Job drawing, mm, ordinate dimensions from the low corner. One solid piece. A direction names the side the tool comes from. Give positions to 0.01 mm unless a question says otherwise; leave off trailing zeros. Order: outer loops, then holes, each group sorted by start corner. A loop starts at its lowest first (then second) coordinate and runs counter-clockwise, first axis right, second up. Notation, with made-up numbers: (80, 40.25) - (101, 40.25) arc R26 ccw to (101, 67.25) - close; hole circle Ø7 at (48.5, 19). An arc over 180 degrees is marked (long way). One line per item, written item: value.
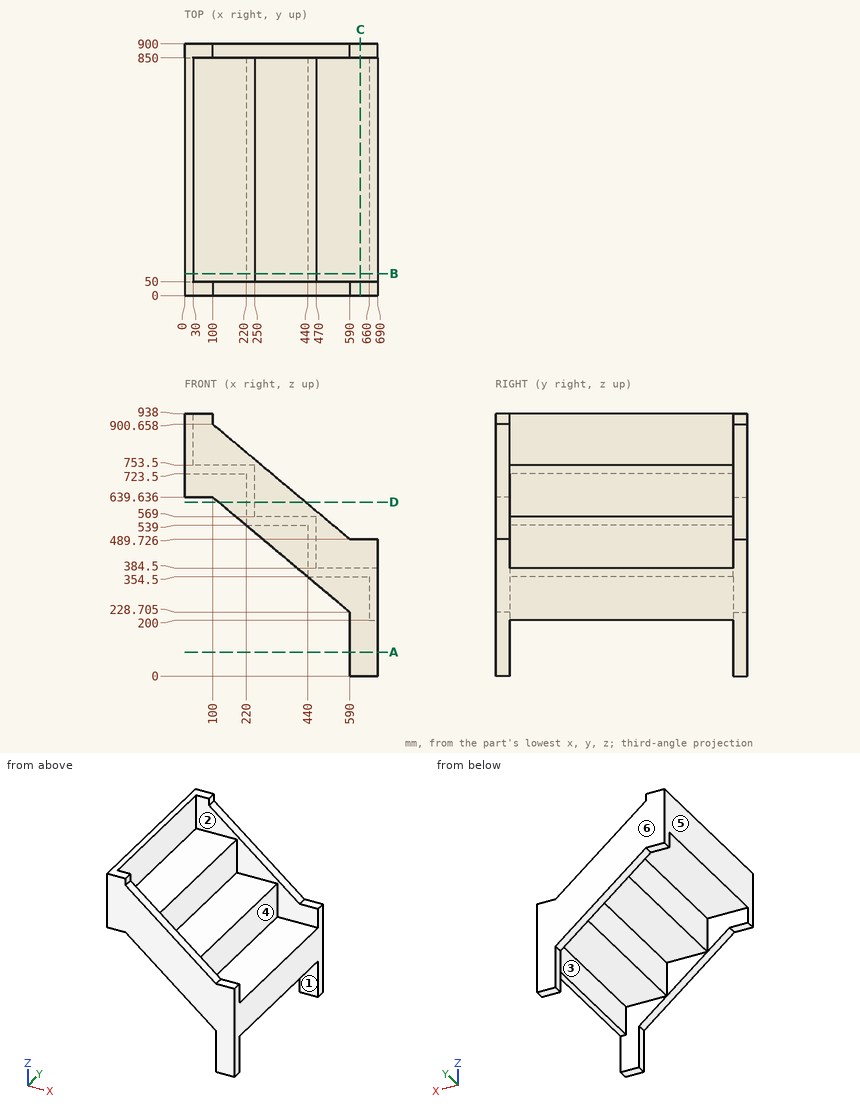
1) Slice it at A-A on z = 85.5. Write the cut outline in (x, y), then the cut area to 3 significant figures.
Answer:
outline: (590, 0) - (690, 0) - (690, 50) - (590, 50) - close; (590, 850) - (690, 850) - (690, 900) - (590, 900) - close
area: 10,000 mm2
2) Wall check: line 1 along Y through (x, z) = (495, 324); line 2 along X through (y, z) = (655, 532.5); line 3 along Z through (x, y) = (513, 498). Give the ranges that are in metal, low to high. Write a range as [from, to].
Answer:
line 1: y = [0, 50], [850, 900]
line 2: x = [440, 470]
line 3: z = [354.5, 384.5]
3) Two-plate mould, pull along Y, no slides. Class the marked faces 3, 4, 5 and 6: pulls with the +Y half, pulls with the -Y half, needs draft (parallel to the pull), parting line crosses it, or undercut.
Answer:
face 3: undercut
face 4: undercut
face 5: needs draft
face 6: pulls with the +Y half
4) Drop flat-ended pins along their axis: P1, Ø6, axis at y = 670.5, z = 767, coming from the +X side; P2, Ø8, axis at y = 494.5, z = 478.5, coming from the +X side; P3, Ø25, axis at x = 615, y = 36, coming from the +Z side. Give the stop position or say it passes through.
Answer:
P1: stops at x = 30
P2: stops at x = 470
P3: stops at z = 489.73
5) Slice it at B-B on y = 79. Write the cut outline in (x, z), then the cut area to 3 significant figures.
Answer:
outline: (0, 723.5) - (220, 723.5) - (220, 539) - (440, 539) - (440, 354.5) - (660, 354.5) - (660, 200) - (690, 200) - (690, 384.5) - (470, 384.5) - (470, 569) - (250, 569) - (250, 753.5) - (30, 753.5) - (30, 938) - (0, 938) - close
area: 41,900 mm2
6) Slice it at C-C on x = 628. Write the cut outline in (y, z), then the cut area to 3 significant figures.
Answer:
outline: (0, 0) - (50, 0) - (50, 354.5) - (850, 354.5) - (850, 0) - (900, 0) - (900, 489.73) - (850, 489.73) - (850, 384.5) - (50, 384.5) - (50, 489.73) - (0, 489.73) - close
area: 73,000 mm2
7) Which spindle directions (+Z, -Z, +X, -X, +Y, -Y) get a long thin tool onto all of the face, cutting with end or side? Do the marked faces 1 and 2. Say none if no direction does.
Answer:
face 1: -Z, -X
face 2: +Z, +X
8) Slice it at D-D on z = 621.5. Write the cut outline in (x, y), then the cut area to 3 significant figures.
Answer:
outline: (121.63, 0) - (432.87, 0) - (432.87, 50) - (250, 50) - (250, 850) - (432.87, 850) - (432.87, 900) - (121.63, 900) - (121.63, 850) - (220, 850) - (220, 50) - (121.63, 50) - close
area: 55,100 mm2
